Drawing for the job (mm, zero at the part's lowest x, y, z). Round coordinates to 2 decimals unless told otherwise and drop trailing zeros. Loops run counter-clockwise (first coordinate to the right, second up) from the corner with the lowest first, then second, coordinate; pieces in that order, holes last. Notation, with made-up numbers: M 78,34.5 L 92,34.5 A4 ccw 92,40.5 Z; hole C -39.75,42 d9. An arc over 180 degrees is marked long. Answer in a Markdown table with one row per item.
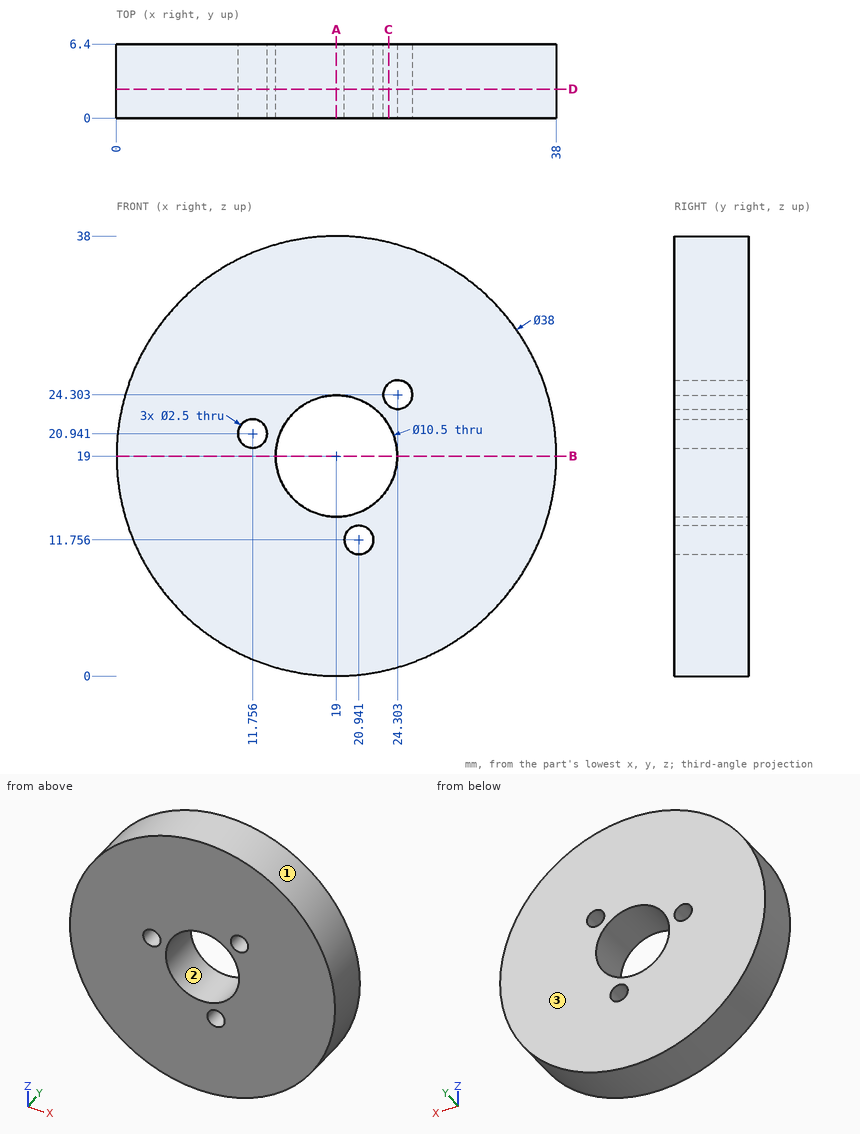
1. Saw through at B-B (z = 19). Write the cut outline in (x, y).
Verdict:
| item | result |
|---|---|
| outline | M 0,0 L 13.75,0 L 13.75,6.4 L 0,6.4 Z; M 24.25,0 L 38,0 L 38,6.4 L 24.25,6.4 Z |
2. Saw through at C-C (x = 23.5). Write the cut outline in (y, z) (1 decimal).
Verdict:
| item | result |
|---|---|
| outline | M 0,0.5 L 6.4,0.5 L 6.4,16.3 L 0,16.3 Z; M 0,21.7 L 6.4,21.7 L 6.4,23.3 L 0,23.3 Z; M 0,25.3 L 6.4,25.3 L 6.4,37.5 L 0,37.5 Z |
3. Pin check, flat tips, straight feed: pin 1 (1 mm diameter, centred on x = 26.5, z = 6, fed in from -Y); pin 2 (1 mm diameter, centred on x = 29, y = 4.5, fed in from -Z) (1 decimal); pin 3 (2 mm diameter, centred on y = 1.5, z = 30.5, fed in from +X) (1 decimal); pin 4 (2 mm diameter, centred on x = 24.3, z = 24.3, fed in from +Y). Stop position of each tip, or through.
Verdict:
| item | result |
|---|---|
| pin 1 | stops at y = 0 |
| pin 2 | stops at z = 2.5 |
| pin 3 | stops at x = 34.8 |
| pin 4 | passes through |
4. Wall check: probe 1 along X at (y, z) = (1.25, 23.5) (1 decimal); probe 2 along X at (y, z) = (2.25, 21.5) (1 decimal); probe 3 along X at (y, z) = (3.75, 23) (1 decimal). Give the ranges that are in metal, low to high.
Verdict:
| item | result |
|---|---|
| probe 1 | x = 0.5 to 16.3, 21.7 to 23.3, 25.3 to 37.5 |
| probe 2 | x = 0.2 to 10.6, 12.9 to 14.4, 23.6 to 37.8 |
| probe 3 | x = 0.4 to 15.6, 22.4 to 37.6 |
5. Saw through at A-A (x = 19). Write the cut outline in (y, z), and give its area (3 significant figures).
Verdict:
| item | result |
|---|---|
| outline | M 0,0 L 6.4,0 L 6.4,13.75 L 0,13.75 Z; M 0,24.25 L 6.4,24.25 L 6.4,38 L 0,38 Z |
| area | 176 mm² |
6. Mould opens along X. For the marked faces 1, 2 and 3 say: +X half, -X half, draft (parallel to the pull), parting line (faces both ways), or undercut.
Verdict:
| item | result |
|---|---|
| face 1 | parting line |
| face 2 | undercut |
| face 3 | draft |
7. Saw through at D-D (y = 2.5). State how many separate pieces and enclosed holes the cut face has, and give its area (3 significant figures).
Verdict:
| item | result |
|---|---|
| separate pieces | 1 |
| enclosed holes | 4 |
| area | 1,030 mm² |
